Could you check a few things on this model? Use its own coordinates, in mm. Give positions to 0.01 mm unless a question says otherwise; leave off trailing zeros. Order: outer loops, then holes, each group sorted by start corner. A loop starts at its lowest first (then second) coordinate and runs counter-clockwise, first axis right, second up. Notation, with made-up numbers: M 58.5,5 L 102.5,5 A24 ccw 102.5,44 Z; hole C 62,76 d8. An arc over 180 degrees is marked long. Use a Markdown table: item, result. Add a question column.
Item 1: If I drill on L1, parallel to Y at x = 52, z = 4; L2, parallel to Z at x = 17.5, y = 156.19 (3 decimals); L3, parallel to Y at x = -59.5, z = 3.25, over which ranges is the centre line in solid material (lowest first)? Write a range as from..to.
Item 2: Suppose I cut it at A-A on z = 3.81. Write out the boundary of the cut face in (x, y) (3 decimals).
Item 3: I'm going to push a flat-ended pin straight in: pin 1 Ø2.5 at (y, z) = (156.19, 3.81) entering from -X. Where does the tip first touch, or does it pass through?
from build123d import *

# Parameters (mm, degrees)
F0_W     = 140
F0_H     = 320
F1_DEPTH = 7.62
F4_R     = 1.905
F5_DEPTH = 140
F3_R     = 1.905
F6_DEPTH = 140


with BuildPart() as f1:
    # F0 (on Top) → F1 (new body)
    with BuildSketch(Plane.XY):
        Rectangle(F0_W, F0_H)
    extrude(amount=F1_DEPTH)

    # F4 (on face) → F5 (cut)
    with BuildSketch(Plane(origin=(-70, 0, 0), x_dir=(0, -1, 0), z_dir=(-1, 0, 0))):
        with Locations((-156.19, 3.81)):
            Circle(F4_R)
    extrude(amount=-F5_DEPTH, mode=Mode.SUBTRACT)

    # F3 (on face) → F6 (cut)
    with BuildSketch(Plane(origin=(-70, 0, 0), x_dir=(0, -1, 0), z_dir=(-1, 0, 0))):
        with Locations((156.19, 3.81)):
            Circle(F3_R)
    extrude(amount=-F6_DEPTH, mode=Mode.SUBTRACT)


solid = f1.part
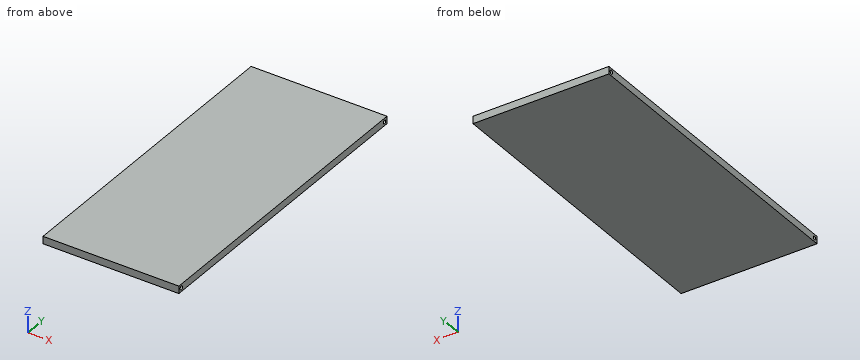
Findings below:
| question | item | result |
|---|---|---|
| 1 | L1 | y = -160..-158.09, -154.29..154.29, 158.09..160 |
| 1 | L2 | z = 0..1.905, 5.715..7.62 |
| 1 | L3 | y = -160..-158.01, -154.37..154.37, 158.01..160 |
| 2 | outline | M -70,-160 L 70,-160 L 70,-158.095 L -70,-158.095 Z; M -70,-154.285 L 70,-154.285 L 70,154.285 L -70,154.285 Z; M -70,158.095 L 70,158.095 L 70,160 L -70,160 Z |
| 3 | pin 1 | passes through |
